```python
from build123d import *

# Parameters (mm, degrees)
SKETCH2_R                                = 36.195
BOSS_EXTRUDE1_DEPTH                      = 10.16
SKETCH3_R                                = 19.05
CUT_EXTRUDE1_DEPTH                       = 11.16
CBORE_FOR_1_4_HEX_HEAD_BOLT1_D           = 6.7564
CBORE_FOR_1_4_HEX_HEAD_BOLT1_CBORE_D     = 11.43
CBORE_FOR_1_4_HEX_HEAD_BOLT1_CBORE_DEPTH = 7.62
CIRPATTERN1_COUNT                        = 6
CIRPATTERN5_COUNT                        = 8
CUT_EXTRUDE9_DEPTH                       = 11.16
F_8_32_TAPPED_HOLE3_D                    = 3.4544


with BuildPart() as part:
    # Sketch2 → Boss-Extrude1 (new body)
    with BuildSketch(Plane.XY):
        Circle(SKETCH2_R)
    extrude(amount=BOSS_EXTRUDE1_DEPTH)

    # Sketch3 → Cut-Extrude1 (cut, through all)
    with BuildSketch(Plane.XY.offset(10.16)):
        Circle(SKETCH3_R)
    extrude(amount=-CUT_EXTRUDE1_DEPTH, mode=Mode.SUBTRACT)

    # CBORE for 1_4 Hex Head Bolt1 (through all)
    with Locations(Plane.XY.offset(10.16)):
        with Locations((0, 29.3624)):
            cbore_for_1_4_hex_head_bolt1 = CounterBoreHole(CBORE_FOR_1_4_HEX_HEAD_BOLT1_D / 2, CBORE_FOR_1_4_HEX_HEAD_BOLT1_CBORE_D / 2, CBORE_FOR_1_4_HEX_HEAD_BOLT1_CBORE_DEPTH)

    # CirPattern1: CBORE for 1_4 Hex Head Bolt1 ×6 about axis
    cirpattern1_axis = Axis((0, 0, 0), (0, 0, 1))
    for i in range(1, CIRPATTERN1_COUNT):
        add(cbore_for_1_4_hex_head_bolt1.rotate(cirpattern1_axis, i * 360 / CIRPATTERN1_COUNT), mode=Mode.SUBTRACT)

    # Sketch35 → 4-40 Tapped Hole1 (revolve, cut)
    with BuildSketch(Plane(origin=(5.465977373, 20.39930527, 10.16), x_dir=(0, -1, 0), z_dir=(1, 0, 0))):
        Polygon((0, 0), (0, 8.299152758), (1.1303, 7.62), (1.1303, 0), align=None)
    f_4_40_tapped_hole1 = revolve(axis=Axis((5.465977373, 20.39930527, 16.51), (0, 0, -1)), mode=Mode.SUBTRACT)

    # CirPattern5: 4-40 Tapped Hole1 ×8 about axis
    cirpattern5_axis = Axis((0, 0, 0), (0, 0, 1))
    for i in range(1, CIRPATTERN5_COUNT):
        add(f_4_40_tapped_hole1.rotate(cirpattern5_axis, i * 360 / CIRPATTERN5_COUNT), mode=Mode.SUBTRACT)

    # Sketch44 → Cut-Extrude9 (cut, through all)
    with BuildSketch(Plane.XY.offset(10.16)):
        Polygon((0, 0), (22.496225018, 38.964604709), (25.245855675, 37.377104709), (2.749630657, -1.5875), align=None)
    extrude(amount=-CUT_EXTRUDE9_DEPTH, mode=Mode.SUBTRACT)

    # 8-32 Tapped Hole3 (through all)
    with Locations(Plane(origin=(-35.885346757, -4.724395527, 5.08), x_dir=(0.130526192, -0.991444861, 0), z_dir=(-0.991444861, -0.130526192, 0))):
        with Locations((0, 0)):
            Hole(F_8_32_TAPPED_HOLE3_D / 2)


solid = part.part
```
Input: part model. Units: mm. Frame: model coordinates. A direction names the side the tool comes from. Give positions to 0.01 mm unless a question says otherwise; leave off trailing zeros. Order: outer loops, then holes, each group sorted by start corner. A loop starts at its lowest first (then second) coordinate and runs counter-clockwise, first axis right, second up. Notation, with made-up numbers: (-27, -23) -> (10, -23) arc R35 ccw to (10, 10) -> close; hole circle Ø1 at (13.5, -17). An arc over 180 degrees is marked (long way). Write each question's results on one line, items separated by ' | '. Start each with the question number.
Item 1: Cut plane A-A on x = 0. Return the cut outline in (y, z) (3 decimals).
Item 2: Mould query, pull axis X, two halves, no side actions, for faces 3 (the flat face through (16, -16, 0)), 4 (the conical face through (10.469, -18.115, 1.979)). Classes: pulls with the +X half, pulls with the -X half, needs draft (parallel to the pull), parting line crosses it, or undercut.
Item 3: Cut plane C-C on x = -14. Return the cut outline in (y, z), then the cut area to 3 significant figures.
Item 4: Cut plane B-B on y = -27. Return the cut outline in (x, z), then the cut area to 3 significant figures.
Item 5: Cut plane D-D on x = 14. Return the cut outline in (y, z).
Item 6: Set-up query: faces 1 (the cylindrical face through (22.206, -13.666, 1.252)), 2 (the cylindrical face through (18.63, 9.48, 6.4)). Return all of +Z, -Z, +X, -X, +Y, -Y with unobstructed straight access to the full face (end or side cutting, diameter ignored); none if empty.
Item 7: Contact query for flat-ended pins moving along their axis: P1, Ø5.5, axis at x = -25.43, y = 14.68, coming from the -Z side; P2, Ø3, axis at y = 6, z = 7, coming from the +X side; P3, Ø1.5, axis at y = -22, z = 8.5, coming from the +X side; P4, Ø5.5, axis at x = 27, y = -17, coming from the +Z side. Output: stop coordinate, or through.
Item 8: Line query: line 1 (Y direction, x = -19.5, z = 4); line 2 (Y direction, x = -1, z = 5.5); line 3 (Z direction, x = 29, y = 4). Output: solid intervals per line, ascending.
Established:
1) outline: (-36.195, 0) -> (-32.741, 0) -> (-32.741, 2.54) -> (-35.077, 2.54) -> (-35.077, 10.16) -> (-36.195, 10.16) -> close; (-25.984, 0) -> (-19.05, 0) -> (-19.05, 10.16) -> (-23.647, 10.16) -> (-23.647, 2.54) -> (-25.984, 2.54) -> close; (19.05, 0) -> (25.984, 0) -> (25.984, 2.54) -> (23.647, 2.54) -> (23.647, 10.16) -> (19.05, 10.16) -> close; (32.741, 0) -> (36.195, 0) -> (36.195, 10.16) -> (35.077, 10.16) -> (35.077, 2.54) -> (32.741, 2.54) -> close
2) face 3: needs draft | face 4: undercut
3) outline: (-33.38, 0) -> (-12.92, 0) -> (-12.92, 10.16) -> (-33.38, 10.16) -> close; (12.92, 0) -> (33.38, 0) -> (33.38, 10.16) -> (12.92, 10.16) -> close | area: 416 mm^2
4) outline: (-24.11, 0) -> (-2.41, 0) -> (-2.41, 2.54) -> (-5.2, 2.54) -> (-5.2, 10.16) -> (-24.11, 10.16) -> close; (2.41, 0) -> (24.11, 0) -> (24.11, 10.16) -> (5.2, 10.16) -> (5.2, 2.54) -> (2.41, 2.54) -> close | area: 398 mm^2
5) outline: (-33.38, 0) -> (-12.92, 0) -> (-12.92, 10.16) -> (-33.38, 10.16) -> close; (12.92, 0) -> (17.9, 0) -> (17.9, 10.16) -> (12.92, 10.16) -> close; (24.25, 0) -> (33.38, 0) -> (33.38, 10.16) -> (24.25, 10.16) -> close
6) face 1: +Z, -Z | face 2: +Z
7) P1: through | P2: x = 35.91 | P3: x = 29.3 | P4: z = 2.54
8) line 1: -30.49 to -3.93, -1.21 to 4.78, 6.15 to 30.49 | line 2: -36.18 to -34.99, -23.74 to -19.02, 19.02 to 23.74, 34.99 to 36.18 | line 3: 0 to 3.36, 6.8 to 10.16
